```python
from build123d import *

# Parameters (mm, degrees)
F0_R     = 9.41
F0_R_2   = 2.405
F1_DEPTH = 10.75


with BuildPart() as f1:
    # F0 (on Top) → F1 (new body)
    with BuildSketch(Plane.XY):
        with BuildLine():
            ThreePointArc((-1.65, 36.752981), (-25.424404, -26.591423), (36.79, 0))
            ThreePointArc((36.79, 0), (26.591423, 25.424404), (1.65, 36.752981))
            Line((1.65, 36.752981), (1.65, 34.1))
            Line((1.65, 34.1), (0, 34.1))
            Line((0, 34.1), (-1.65, 34.1))
            Line((-1.65, 34.1), (-1.65, 36.752981))
        make_face()
        with Locations((-13.007229, -13.007229)):
            Circle(F0_R, mode=Mode.SUBTRACT)
        with Locations((13.007229, -13.007229)):
            Circle(F0_R, mode=Mode.SUBTRACT)
        with Locations((-13.007229, 13.007229)):
            Circle(F0_R, mode=Mode.SUBTRACT)
        Circle(F0_R_2, mode=Mode.SUBTRACT)
        with Locations((13.007229, 13.007229)):
            Circle(F0_R, mode=Mode.SUBTRACT)
    extrude(amount=F1_DEPTH)


solid = f1.part
```
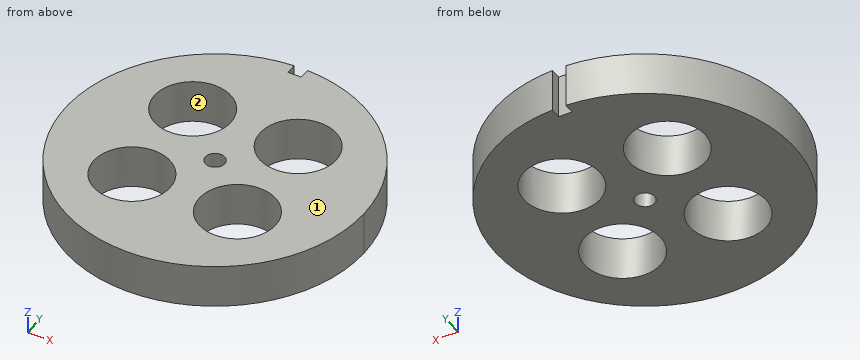
CAD build for the part. Positions are in the model's coordinates, mm. Face numbers are marked on the shaded views. Round coordinates to 2 decimals unless told otherwise and drop trailing zeros. Loops run counter-clockwise (first coordinate to the right, second up) from the corner with the lowest first, then second, coordinate; pieces in that order, holes last. Notation, with made-up numbers: M 46,65 L 95,65 A20 cw 95,79 Z; hole C 46.25,19.5 d6. An arc over 180 degrees is marked long. Use a Markdown table: item, result. Add a question column.
(1) Drill centre lines: line 1 (Y direction, x = -20, z = 4.5); line 2 (X direction, y = 15.5, z = 0.5); line 3 (Y direction, x = 6, z = 3.75). Where is each one in solid material? Low to high.
(2) Cut at B-B (y = -17). Give the cut face in (x, z), and give its area (3 significant figures).
(3) Cut at C-C (z = 1.25). Give the cut face in (x, y) (3 decimals).
(4) Cut at D-D (x = -10.5). Give the cut face in (y, z), and give its area (3 significant figures).
(5) Flat gauge pins, fed straight in: pin 1 (1 mm diameter, centred on x = -1, z = 4, fed in from -Y); pin 2 (2 mm diameter, centred on y = -17.5, z = 3.5, fed in from -X); pin 3 (4 mm diameter, centred on y = -24, z = 1.5, fed in from -X). Where does each tip first touch, or does it go through?
(6) Cut at A-A (x = 0). Give the cut face in (y, z) (3 decimals).
(7) Pull direction X, two halves, no side cores. Call the marked faces 1 and 2: +X half, -X half, draft (parallel to the pull), parting line (faces both ways), or undercut.
Geometry says:
| question | item | result |
|---|---|---|
| 1 | line 1 | y = -30.88 to -19.3, -6.71 to 6.71, 19.3 to 30.88 |
| 1 | line 2 | x = -33.37 to -22.08, -3.93 to 3.93, 22.08 to 33.37 |
| 1 | line 3 | y = -36.3 to -19.29, -6.73 to 6.73, 19.29 to 36.3 |
| 2 | outline | M -32.63,0 L -21.53,0 L -21.53,10.75 L -32.63,10.75 Z; M -4.49,0 L 4.49,0 L 4.49,10.75 L -4.49,10.75 Z; M 21.53,0 L 32.63,0 L 32.63,10.75 L 21.53,10.75 Z |
| 2 | area | 335 mm² |
| 3 | outline | M -1.65,34.1 L -1.65,36.753 A36.79 ccw long 1.65,36.753 L 1.65,34.1 Z; hole C -13.007,-13.007 d18.82; hole C -13.007,13.007 d18.82; hole C 0,0 d4.81; hole C 13.007,-13.007 d18.82; hole C 13.007,13.007 d18.82 |
| 4 | outline | M -35.26,0 L -22.08,0 L -22.08,10.75 L -35.26,10.75 Z; M -3.94,0 L 3.94,0 L 3.94,10.75 L -3.94,10.75 Z; M 22.08,0 L 35.26,0 L 35.26,10.75 L 22.08,10.75 Z |
| 4 | area | 368 mm² |
| 5 | pin 1 | stops at y = -36.79 |
| 5 | pin 2 | stops at x = -32.88 |
| 5 | pin 3 | stops at x = -29.49 |
| 6 | outline | M -36.79,0 L -2.405,0 L -2.405,10.75 L -36.79,10.75 Z; M 2.405,0 L 34.1,0 L 34.1,10.75 L 2.405,10.75 Z |
| 7 | face 1 | draft |
| 7 | face 2 | undercut |
